Verification items for the finished model (mm, model axes). Round coordinates to 2 decimals unless told otherwise and drop trailing zeros. Order: outer loops, then holes, each group sorted by start corner. A loop starts at its lowest first (then second) coordinate and runs counter-clockwise, first axis right, second up. Notation, with made-up numbers: (66.25, -20) -> (101.25, -20) arc R27 cw to (101.25, -2) -> close; hole circle Ø2 at (-15, 20.5). An arc over 180 degrees is marked (long way). Put each result on its own line as item: value.
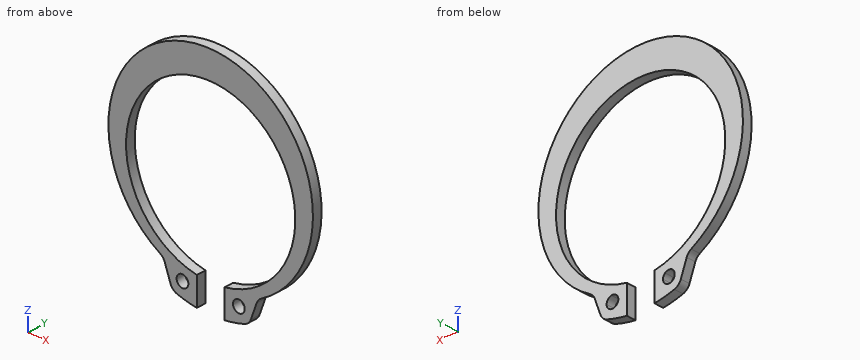
```python
from build123d import *

# Parameters (mm, degrees)
F1_DEPTH = 2
F2_R     = 2.15


# Not quite as in the source:
# - a feature names something its author has since deleted; it is built from what else it names


with BuildPart() as f1:
    # F0 (on Front) → F1 (new body)
    with BuildSketch(Plane.XZ):
        with BuildLine():
            ThreePointArc((-2.95, -17.7566184844), (0, 18), (2.95, -17.7566184844))
            Line((2.95, -17.7566184844), (2.95, -19.4990138986))
            ThreePointArc((2.95, -19.4990138986), (4.0741879212, -19.3150062668), (5.1871999415, -19.0723923069))
            ThreePointArc((5.1871999415, -19.0723923069), (5.6730323101, -18.8149936793), (6.2223129211, -18.7909529991))
            ThreePointArc((6.2223129211, -18.7909529991), (8.1825487808, -18.102131288), (10.0681136131, -17.2294084005))
            ThreePointArc((10.0681136131, -17.2294084005), (0, 23.8), (-10.0681136131, -17.2294084005))
            ThreePointArc((-10.0681136131, -17.2294084005), (-8.1825487808, -18.102131288), (-6.2223129211, -18.7909529991))
            ThreePointArc((-6.2223129211, -18.7909529991), (-5.6730323101, -18.8149936793), (-5.1871999415, -19.0723923069))
            ThreePointArc((-5.1871999415, -19.0723923069), (-4.0741879212, -19.3150062668), (-2.95, -19.4990138986))
            Line((-2.95, -19.4990138986), (-2.95, -17.7566184844))
        make_face()
        with BuildLine():
            ThreePointArc((5.1871999415, -19.0723923069), (4.0741879212, -19.3150062668), (2.95, -19.4990138986))
            Line((2.95, -19.4990138986), (2.95, -23.6566184844))
            ThreePointArc((2.95, -23.6566184844), (5.6060820605, -23.1713172273), (8.1902527715, -22.3887886599))
            Line((8.1902527715, -22.3887886599), (10.0681136131, -17.2294084005))
            ThreePointArc((10.0681136131, -17.2294084005), (8.1825487808, -18.102131288), (6.2223129211, -18.7909529991))
            ThreePointArc((6.2223129211, -18.7909529991), (6.9599367667, -19.2193782076), (7.2509916054, -20.0212037359))
            ThreePointArc((7.2509916054, -20.0212037359), (5.4788515763, -21.1569280818), (5.1871999415, -19.0723923069))
        make_face()
        with BuildLine():
            Line((-2.95, -23.6566184844), (-2.95, -19.4990138986))
            ThreePointArc((-2.95, -19.4990138986), (-4.0741879212, -19.3150062668), (-5.1871999415, -19.0723923069))
            ThreePointArc((-5.1871999415, -19.0723923069), (-4.8652672595, -19.4990637067), (-4.7509916054, -20.0212037359))
            ThreePointArc((-4.7509916054, -20.0212037359), (-6.8028171337, -20.9801488971), (-6.2223129211, -18.7909529991))
            ThreePointArc((-6.2223129211, -18.7909529991), (-8.1825487808, -18.102131288), (-10.0681136131, -17.2294084005))
            Line((-10.0681136131, -17.2294084005), (-8.1902527715, -22.3887886599))
            ThreePointArc((-8.1902527715, -22.3887886599), (-5.6060820605, -23.1713172273), (-2.95, -23.6566184844))
        make_face()
    extrude(amount=F1_DEPTH)

    # F2
    f2_edges = [f1.edges().sort_by_distance(p)[0] for p in [
        (-10.068114, -1, -17.229408),
        (-8.190253, -1, -22.388789),
        (8.190253, -1, -22.388789),
        (10.068114, -1, -17.229408),
    ]]
    fillet(f2_edges, radius=F2_R)


solid = f1.part
```
Item 1: Sectioned sample at C-C, the plane x = 13. Record the boundary of the cut face in (y, z), then the cut area to 4 significant figures.
Geometry check:
outline: (-2, -15.39) -> (0, -15.39) -> (0, -12.45) -> (-2, -12.45) -> close; (-2, 12.45) -> (0, 12.45) -> (0, 19.49) -> (-2, 19.49) -> close
area: 19.95 mm2
Item 2: Sectioned sample at D-D, the plane x = 0. Record the boundary of the cut face in (y, z), then the cut area to 3 significant figures.
Geometry check:
outline: (-2, 18) -> (0, 18) -> (0, 23.8) -> (-2, 23.8) -> close
area: 11.6 mm2
Item 3: Depth check by flat-ended pin: pin 1 Ø4 at (x, z) = (-6, -20.02) entering from +Y. Enter the tip coordinate at first touch or a pass-through.
Geometry check:
pin 1: y = 0
Item 4: Material ranges on line 1 along Z through (x, y) = (0, -0.85); line 2 along X through (y, z) = (-1.4, 15.5); line 3 along Z through (x, y) = (5, -0.4), recorded low to high.
Geometry check:
line 1: 18 to 23.8
line 2: -17.09 to -9.15, 9.15 to 17.09
line 3: -23.31 to -20.77, -19.27 to -17.29, 17.29 to 23.22
Item 5: Sectioned sample at B-B, the plane z = -9. Record the boundary of the cut face in (x, y), then the cut area to 3 significant figures.
Geometry check:
outline: (-18.73, -2) -> (-15.59, -2) -> (-15.59, 0) -> (-18.73, 0) -> close; (15.59, -2) -> (18.73, -2) -> (18.73, 0) -> (15.59, 0) -> close
area: 12.6 mm2
Item 6: Sectioned sample at A-A, the plane y = -0.9. Record the boundary of the cut face in (x, z), then the cut area to 3 significant figures.
Geometry check:
outline: (-10.75, -16.86) arc R2.15 cw to (-9.79, -17.99) -> (-8.54, -21.42) arc R2.15 ccw to (-7.17, -22.74) arc R23.84 ccw to (-2.95, -23.66) -> (-2.95, -17.76) arc R18 cw (long way) to (2.95, -17.76) -> (2.95, -23.66) arc R23.84 ccw to (7.17, -22.74) arc R2.15 ccw to (8.54, -21.42) -> (9.79, -17.99) arc R2.15 cw to (10.75, -16.86) arc R21.75 ccw (long way) to start; hole circle Ø2.5 at (-6, -20.02); hole circle Ø2.5 at (6, -20.02)
area: 500 mm2
